Here's how the part is built. I have some questions about the finished solid (model axes, mm). A direction names the side the tool comes from. Give positions to 0.01 mm unless a question says otherwise; leave off trailing zeros. Loops run counter-clockwise (first coordinate to the right, second up) from the corner with the lowest first, then second, coordinate; pieces in that order, holes last. Notation, with made-up numbers: (-27.75, -0.75) - (-5.75, -0.75) arc R15 ccw to (-5.75, 18.25) - close; hole circle Ø11 at (75.5, 25). An arc over 180 degrees is marked (long way). Use a Markdown table: item, result.
from build123d import *

# Parameters (mm, degrees)
SKETCH1_W           = 8
SKETCH1_H           = 6
SKETCH1_W_2         = 20
SKETCH1_H_2         = 22
BOSS_EXTRUDE1_DEPTH = 30
SKETCH2_W           = 66
SKETCH2_H           = 20.2
CUT_EXTRUDE1_DEPTH  = 22
SKETCH3_W           = 8
SKETCH3_H           = 6
BOSS_EXTRUDE2_DEPTH = 46
FILLET1_R           = 30
FILLET2_R           = 20
FILLET3_R           = 10
FILLET4_R           = 2
FILLET5_R           = 1


with BuildPart() as part:
    # Sketch1 → Boss-Extrude1 (new body)
    with BuildSketch(Plane(origin=(0, 0, 0), x_dir=(1, 0, 0), z_dir=(0, 1, 0))):
        with BuildLine():
            Line((-13, 41), (-33, 41))
            Line((-33, 41), (-33, 6))
            Line((-33, 6), (-32.449961479, 6))
            ThreePointArc((-32.449961479, 6), (0, 33), (32.449961479, 6))
            Line((32.449961479, 6), (33, 6))
            Line((33, 6), (33, 41))
            Line((33, 41), (13, 41))
            Line((13, 41), (-13, 41))
        make_face()
        with Locations((-37, 3)):
            Rectangle(SKETCH1_W, SKETCH1_H)
        with BuildLine():
            Line((-32.449961479, 6), (-33, 6))
            Line((-33, 6), (-33, 0))
            ThreePointArc((-33, 0), (-32.862202671, 3.012579558), (-32.449961479, 6))
        make_face()
        with Locations((37, 3)):
            Rectangle(SKETCH1_W, SKETCH1_H)
        with BuildLine():
            ThreePointArc((32.449961479, 6), (32.862202671, 3.012579558), (33, 0))
            Line((33, 0), (33, 6))
            Line((33, 6), (32.449961479, 6))
        make_face()
        with Locations((-23, 52)):
            Rectangle(SKETCH1_W_2, SKETCH1_H_2)
        with Locations((23, 52)):
            Rectangle(SKETCH1_W_2, SKETCH1_H_2)
    extrude(amount=BOSS_EXTRUDE1_DEPTH)

    # Sketch2 → Cut-Extrude1 (cut)
    with BuildSketch(Plane(origin=(0, 0, -63), x_dir=(-1, 0, 0), z_dir=(0, 0, -1))):
        with Locations((0, 15)):
            Rectangle(SKETCH2_W, SKETCH2_H)
    extrude(amount=-CUT_EXTRUDE1_DEPTH, mode=Mode.SUBTRACT)

    # Sketch3 → Boss-Extrude2 (add)
    with BuildSketch(Plane(origin=(0, 30, 0), x_dir=(1, 0, 0), z_dir=(0, 1, 0))):
        with BuildLine():
            Line((-33, 41), (-33, 6))
            Line((-33, 6), (-32.449961479, 6))
            ThreePointArc((-32.449961479, 6), (0, 33), (32.449961479, 6))
            Line((32.449961479, 6), (33, 6))
            Line((33, 6), (33, 41))
            Line((33, 41), (13, 41))
            Line((13, 41), (-13, 41))
            Line((-13, 41), (-33, 41))
        make_face()
        with Locations((37, 3)):
            Rectangle(SKETCH3_W, SKETCH3_H)
        with Locations((-37, 3)):
            Rectangle(SKETCH3_W, SKETCH3_H)
        with BuildLine():
            Line((-32.449961479, 6), (-33, 6))
            Line((-33, 6), (-33, 0))
            ThreePointArc((-33, 0), (-32.862202671, 3.012579558), (-32.449961479, 6))
        make_face()
        with BuildLine():
            Line((33, 6), (32.449961479, 6))
            ThreePointArc((32.449961479, 6), (32.862202671, 3.012579558), (33, 0))
            Line((33, 0), (33, 6))
        make_face()
    extrude(amount=BOSS_EXTRUDE2_DEPTH)

    # Fillet1
    # the kernel refuses this fillet: 30 mm, written as the material it adds along each edge
    with BuildSketch(Plane(origin=(59.284161474, 30, -41), x_dir=(0, 1, 0), z_dir=(-1, 0, 0))) as fillet1_piece_1_section:
        with BuildLine():
            CenterArc((28.91366459, 30), FILLET1_R, 195.466009953, 74.533990047)
            Line((0, 22), (-0.578273292, 21.84))
            ThreePointArc((-0.578273292, 21.84), (-0.6, 11), (-0.6, 0))
            Line((-0.6, 0), (0, -0.6))
            Line((0, -0.6), (28.91366459, -0.6))
            Line((28.91366459, -0.6), (28.91366459, 0))
        make_face()
    fillet1_piece_1 = extrude(amount=92.284161474, mode=Mode.PRIVATE)
    fillet1_piece_1 = split(fillet1_piece_1, bisect_by=Plane(origin=(33, 36.836030265, -46.582233156), z_dir=(-1, 0, 0)), keep=Keep.TOP, mode=Mode.PRIVATE)
    fillet1_piece_1 = split(fillet1_piece_1, bisect_by=Plane(origin=(13, 36.836030265, -46.582233156), z_dir=(1, 0, 0)), keep=Keep.TOP, mode=Mode.PRIVATE)
    add(fillet1_piece_1)
    with BuildSketch(Plane(origin=(-13, 30, -41), x_dir=(0, 1, 0), z_dir=(-1, 0, 0)), Plane(origin=(33, 30, -41), x_dir=(0, 1, 0), z_dir=(-1, 0, 0))) as fillet1_piece_2:
        with BuildLine():
            CenterArc((28.91366459, 30), FILLET1_R, 195.466009953, 74.533990047)
            Line((0, 22), (-0.578273292, 21.84))
            ThreePointArc((-0.578273292, 21.84), (-0.6, 11), (-0.6, 0))
            Line((-0.6, 0), (0, -0.6))
            Line((0, -0.6), (28.91366459, -0.6))
            Line((28.91366459, -0.6), (28.91366459, 0))
        make_face()
    extrude(amount=20)
    with BuildSketch(Plane(origin=(33, 30, -41), x_dir=(0, 1, 0), z_dir=(-1, 0, 0))) as fillet1_piece_3_section:
        with BuildLine():
            CenterArc((28.91366459, 30), FILLET1_R, 195.466009953, 74.533990047)
            Line((0, 22), (-0.578273292, 21.84))
            ThreePointArc((-0.578273292, 21.84), (-0.6, 11), (-0.6, 0))
            Line((-0.6, 0), (0, -0.6))
            Line((0, -0.6), (28.91366459, -0.6))
            Line((28.91366459, -0.6), (28.91366459, 0))
        make_face()
    fillet1_piece_3 = extrude(amount=92.284161474, mode=Mode.PRIVATE)
    fillet1_piece_3 = split(fillet1_piece_3, bisect_by=Plane(origin=(-33, 36.836030265, -46.582233156), z_dir=(1, 0, 0)), keep=Keep.TOP, mode=Mode.PRIVATE)
    fillet1_piece_3 = split(fillet1_piece_3, bisect_by=Plane(origin=(-13, 36.836030265, -46.582233156), z_dir=(-1, 0, 0)), keep=Keep.TOP, mode=Mode.PRIVATE)
    add(fillet1_piece_3)

    # Fillet2
    # the kernel refuses this fillet: 20 mm, written as the material it adds along each edge
    with BuildSketch(Plane(origin=(33, 76, -6), x_dir=(0, 0, -1), z_dir=(0, -1, 0)), Plane(origin=(-33, 0, -6), x_dir=(0, 0, -1), z_dir=(0, 1, 0))) as fillet2_piece_1:
        with BuildLine():
            CenterArc((16, 20), FILLET2_R, 216.869897646, 53.130102354)
            Line((0, 8), (-0.32, 7.76))
            ThreePointArc((-0.32, 7.76), (-0.4, 4), (-0.4, 0))
            Line((-0.4, 0), (0, -0.4))
            Line((0, -0.4), (16, -0.4))
            Line((16, -0.4), (16, 0))
        make_face()
    extrude(amount=76)

    # Fillet3
    fillet3_edges = [part.edges().sort_by_distance(p)[0] for p in [
        (-13, 42.006832295, -41),
        (13, 2.45, -41),
        (13, 42.006832295, -41),
        (-13, 2.45, -41),
    ]]
    fillet(fillet3_edges, radius=FILLET3_R)

    # Fillet4
    fillet4_edges = [part.edges().sort_by_distance(p)[0] for p in [
        (-23, 25.1, -63),
        (-23, 4.9, -63),
        (23, 25.1, -63),
        (23, 4.9, -63),
    ]]
    fillet(fillet4_edges, radius=FILLET4_R)

    # Fillet5
    fillet5_edges = [part.edges().sort_by_distance(p)[0] for p in [
        (-18, 25.1, -41),
        (-18, 4.9, -41),
        (18, 25.1, -41),
        (18, 4.9, -41),
    ]]
    fillet(fillet5_edges, radius=FILLET5_R)


solid = part.part
(1) Suppose I cut it at D-D on x = -6. Write out the boundary of the cut face in (y, z), plus the area to 3 significant figures.
A:
| item | result |
|---|---|
| outline | (0, -41.46) - (5.06, -41.46) arc R1 cw to (5.9, -41) - (24.1, -41) arc R1 cw to (24.94, -41.46) - (53.68, -41.46) arc R30 cw to (58.91, -41) - (76, -41) - (76, -32.45) - (0, -32.45) - close |
| area | 666 mm2 |
(2) If I drill on line 1 (X direction, y = 4.5, z = -51.5); line 2 (X direction, y = 22, z = -30); line 3 (Y direction, x = -32.5, z = -54), over which ranges is the centre line in solid material (lowest first)?
A:
| item | result |
|---|---|
| line 1 | -33 to -13, 13 to 33 |
| line 2 | -33 to -13.75, 13.75 to 33 |
| line 3 | 0 to 4.9, 25.1 to 34.2 |
(3) We'd pull the mould along X, two halves only. Please class faces 1 (the face through (1, 0, -39)), 2 (the face through (33, 37, -38)), 3 (the face through (13, 2, -57)): pulls with the +X half, pulls with the -X half, needs draft (parallel to the pull), parting line crosses it, or undercut.
A:
| item | result |
|---|---|
| face 1 | needs draft |
| face 2 | pulls with the +X half |
| face 3 | undercut |
(4) Suppose I cut it at B-B on z = -23.5. Write out the boundary of the cut face in (x, y), plus the area to 3 significant figures.
A:
| item | result |
|---|---|
| outline | (-33, 0) - (-23.17, 0) - (-23.17, 76) - (-33, 76) - close; (23.17, 0) - (33, 0) - (33, 76) - (23.17, 76) - close |
| area | 1,490 mm2 |
(5) Will these pins go through, and if not, where does the flat tip stop? pin 1 (3 mm diameter, centred on x = 28, y = 34.5, fed in from -Z); pin 2 (5.5 mm diameter, centred on y = 31, z = -56, fed in from -X); pin 3 (5.5 mm diameter, centred on x = -26.5, z = -51.5, fed in from +Y).
A:
| item | result |
|---|---|
| pin 1 | z = -55.88 |
| pin 2 | x = -33 |
| pin 3 | y = 38.79 |
(6) Suppose I cut it at A-A on z = -46.5. Write out the boundary of the cut face in (x, y).
A:
| item | result |
|---|---|
| outline | (-33, 0) - (-11.93, 0) - (-11.93, 4.9) - (-33, 4.9) - close; (-33, 25.1) - (-11.93, 25.1) - (-11.93, 41.6) - (-33, 41.6) - close; (11.93, 0) - (33, 0) - (33, 4.9) - (11.93, 4.9) - close; (11.93, 25.1) - (33, 25.1) - (33, 41.6) - (11.93, 41.6) - close |
(7) Suppose I cut it at C-C on y = 20.5. Write out the boundary of the cut face in (x, z), plus the area to 3 significant figures.
A:
| item | result |
|---|---|
| outline | (-41, -6) arc R20 cw to (-33, -22) - (-33, -41) - (33, -41) - (33, -22) arc R20 cw to (41, -6) - (41, 0) - (33, 0) arc R33 cw to (-33, 0) - (-41, 0) - close |
| area | 1,170 mm2 |
(8) On a 3-axis mill with a long thin cutter (end or side, diameter ignored), from which of +Z, -Z, +X, -X, +Y, -Y can I reach the whole of each face in a straight line? I mean faces 4 (the face through (0, 37, -41)), 5 (the face through (13, 29, -56)), 6 (the face through (-33, 39, -38)), 7 (the face through (23, 4.9, -52)). Say none if no direction works.
A:
| item | result |
|---|---|
| face 4 | -Z |
| face 5 | -Z, +Y, -Y |
| face 6 | -Z, -X, +Y, -Y |
| face 7 | -Z, +X, -X |
